Autodesk Inventor part; units mm, degrees
ref_plane "YZ Plane" through (0, 0, 0) normal (1, 0, 0) x (0, 1, 0)
ref_plane "XZ Plane" through (0, 0, 0) normal (0, 1, 0) x (-1, 0, 0)
ref_plane "XY Plane" through (0, 0, 0) normal (0, 0, 1) x (1, 0, 0)
sketch "Sketch1" plane through (0, 0, 0) normal (0, 0, 1) x (1, 0, 0)
  line L0 (0, 76.454) -> (0, -76.454)
  line L1 (-57.4294, 0) -> (57.4294, 0)
  line L2 (41.021, -54.61) -> (-41.021, -54.61)
  line L3 (-41.021, -54.61) -> (-41.021, 54.61)
  line L4 (-41.021, 54.61) -> (41.021, 54.61)
  line L5 (41.021, 54.61) -> (41.021, -54.61)
  line L6 (41.021, -54.61) -> (-41.021, 54.61) construction
  line L7 (-41.021, -54.61) -> (41.021, 54.61) construction
  line L8 (15.875, 43.18) -> (-15.875, 43.18) construction
  line L9 (15.875, 48.26) -> (-15.875, 48.26)
  line L10 (-15.875, 38.1) -> (15.875, 38.1)
  arc A0 (15.875, 38.1) -> (15.875, 48.26) centre (15.875, 43.18) ccw
  arc A1 (-15.875, 48.26) -> (-15.875, 38.1) centre (-15.875, 43.18) ccw
  point P0 (0, 0)
  point P1 (0, 43.18)
  dimension "d0" = 82.042
  dimension "d1" = 109.22
  dimension "d4" = 31.75
  dimension "d5" = 6.35
  dimension "d6" = 5.08
extrude "Extrusion1" add sketch "Sketch1" along normal blind 2.9972 contours L4 L5 L1 L0 L10 A0 L9 | L0 L9 A1 L10 L1 L3 L4 | L1 L0 L2 L3 | L5 L2 L0 L1
fillet "Fillet1" radius 3.175 2 edges at (-41.021, 54.61, 1.4986) (41.021, 54.61, 1.4986)
chamfer "Chamfer1" distance 6.35 angle 45 2 edges at (41.021, -54.61, 1.4986) (-41.021, -54.61, 1.4986)
fillet "Fillet2" radius 3.175 4 edges at (-41.021, -48.26, 1.4986) (-34.671, -54.61, 1.4986) (34.671, -54.61, 1.4986) (41.021, -48.26, 1.4986)
properties part number "J010355" material "ACRYLIC, CLEAR"
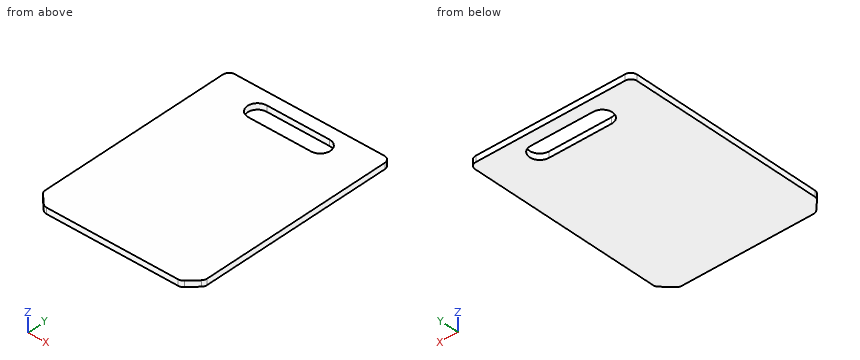
Could you check a few things on this model? Use its own coordinates, in mm. Coordinates: 2 decimals unless noted, no trailing zeros. Write each loop counter-clockwise with the first axis right and the second up, starting at its lowest first coordinate (ties: lowest second). Pieces come first, ordered by that corner, then holes. Notation, with made-up numbers: (3, 32) - (31, 32) arc R15 cw to (31, 57) - close; hole circle Ø1 at (-26, 19). An arc over 180 degrees is marked (long way). Put each result on its own line as item: value. Start each with the question number.
Q1. I want a section at B-B on x = -3. Write out the boundary of the cut face in (y, z), plus the area to 3 significant figures.
Q2. Please list where these lines run through material, in increasing order: L1, parallel to Y at x = -0.5, z = 1.15; L2, parallel to Y at x = 19, z = 1.65; L3, parallel to Y at x = -34, z = 2.2.
Q3. I want a section at C-C on z = 2.25. Write out the boundary of the cut face in (x, y) (3 decimals), plus the area to 3 significant figures.
Q4. I want a section at A-A on y = 43.18. Write out the boundary of the cut face in (x, z) (3 decimals), plus the area to 3 significant figures.
Checks:
1. outline: (-54.61, 0) - (38.1, 0) - (38.1, 3) - (-54.61, 3) - close; (48.26, 0) - (54.61, 0) - (54.61, 3) - (48.26, 3) - close
1. area: 297 mm²
2. L1: -54.61 to 38.1, 48.26 to 54.61
2. L2: -54.61 to 39.17, 47.19 to 54.61
2. L3: -54.54 to 54.61
3. outline: (-41.021, -46.945) arc R3.175 ccw to (-40.091, -49.19) - (-35.601, -53.68) arc R3.175 ccw to (-33.356, -54.61) - (33.356, -54.61) arc R3.175 ccw to (35.601, -53.68) - (40.091, -49.19) arc R3.175 ccw to (41.021, -46.945) - (41.021, 51.435) arc R3.175 ccw to (37.846, 54.61) - (-37.846, 54.61) arc R3.175 ccw to (-41.021, 51.435) - close; hole (-15.875, 38.1) - (15.875, 38.1) arc R5.08 ccw to (15.875, 48.26) - (-15.875, 48.26) arc R5.08 ccw to start
3. area: 8,510 mm²
4. outline: (-41.021, 0) - (-20.955, 0) - (-20.955, 2.997) - (-41.021, 2.997) - close; (20.955, 0) - (41.021, 0) - (41.021, 2.997) - (20.955, 2.997) - close
4. area: 120 mm²
